from build123d import *

# Parameters (mm, degrees)
BOSS_EXTRUDE1_DEPTH = 59.69
SKETCH31_R          = 3.9878
CUT_EXTRUDE1_DEPTH  = 31.226


with BuildPart() as part:
    # Sketch30 → Boss-Extrude1 (new body)
    with BuildSketch(Plane(origin=(0, 0, -44.196), x_dir=(-1, 0, 0), z_dir=(0, 0, -1))):
        with BuildLine():
            Line((-21.122639806, -11.230837818), (-19.351377941, -18.999086285))
            Line((-19.351377941, -18.999086285), (-11.19917043, -18.999086285))
            Line((-11.19917043, -18.999086285), (-11.58017043, -47.00394942))
            Line((-11.58017043, -47.00394942), (-17.42217043, -47.00394942))
            Line((-17.42217043, -47.00394942), (-17.42217043, -26.68394942))
            Line((-17.42217043, -26.68394942), (-17.42217043, -25.349086285))
            ThreePointArc((-17.42217043, -25.349086285), (-25.786020569, -21.520936424), (-29.61417043, -13.157086285))
            Line((-29.61417043, -13.157086285), (-29.61417043, 6.33605058))
            ThreePointArc((-29.61417043, 6.33605058), (-25.894426551, 15.316306701), (-16.91417043, 19.03605058))
            Line((-16.91417043, 19.03605058), (0.10382957, 19.03605058))
            ThreePointArc((0.10382957, 19.03605058), (9.084085691, 15.316306701), (12.80382957, 6.33605058))
            Line((12.80382957, 6.33605058), (12.80382957, -13.157086285))
            ThreePointArc((12.80382957, -13.157086285), (8.975679709, -21.520936424), (0.61182957, -25.349086285))
            Line((0.61182957, -25.349086285), (0.61182957, -26.68394942))
            Line((0.61182957, -26.68394942), (0.61182957, -47.00394942))
            Line((0.61182957, -47.00394942), (-5.23017043, -47.00394942))
            Line((-5.23017043, -47.00394942), (-5.61117043, -18.999086285))
            Line((-5.61117043, -18.999086285), (2.54103708, -18.999086285))
            Line((2.54103708, -18.999086285), (4.312298946, -11.230837818))
            ThreePointArc((4.312298946, -11.230837818), (8.246380302, -8.403768679), (6.679296605, -3.81971319))
            ThreePointArc((6.679296605, -3.81971319), (7.525853874, 2.546365897), (5.417372104, 8.61249537))
            ThreePointArc((5.417372104, 8.61249537), (4.777900298, 13.775697179), (-0.415899, 14.079054992))
            ThreePointArc((-0.415899, 14.079054992), (-8.40517043, 15.22605058), (-16.394441861, 14.079054992))
            ThreePointArc((-16.394441861, 14.079054992), (-21.588241548, 13.775696815), (-22.227712388, 8.612494473))
            ThreePointArc((-22.227712388, 8.612494473), (-24.336184911, 2.546364848), (-23.489636452, -3.819712493))
            ThreePointArc((-23.489636452, -3.819712493), (-25.056721349, -8.403768093), (-21.122639806, -11.230837818))
        make_face()
    extrude(amount=BOSS_EXTRUDE1_DEPTH)

    # Sketch31 → Cut-Extrude1 (cut, through all)
    with BuildSketch(Plane(origin=(17.42217043, 0, 0), x_dir=(0, 0, -1), z_dir=(1, 0, 0))):
        with Locations(Location((95.9104, -36.00574942, 0), (0, 0, 90))):  # turned: the seam where the file's is
            Circle(SKETCH31_R)
        with Locations(Location((70.8914, -36.00574942, 0), (0, 0, 90))):  # turned: the seam where the file's is
            Circle(SKETCH31_R)
        with Locations(Location((54.1782, -38.11394942, 0), (0, 0, 90))):  # turned: the seam where the file's is
            Circle(SKETCH31_R)
    extrude(amount=-CUT_EXTRUDE1_DEPTH, mode=Mode.SUBTRACT)


solid = part.part
The model under review builds one solid part; all positions refer to its coordinate system, in mm. A direction names the side the tool comes from. Coordinates: 2 decimals unless noted, no trailing zeros. Loops run counter-clockwise (first coordinate to the right, second up) from the corner with the lowest first, then second, coordinate; pieces in that order, holes last. Notation, with made-up numbers: (-21.5, -0.5) -> (10.5, -0.5) arc R19 cw to (10.5, 15.5) -> close; hole circle Ø2 at (-19.75, -7.5). An arc over 180 degrees is marked (long way). Use a Markdown table: item, result. Add a question column.
1. To check wall thickness, follow line 1 (X direction, y = -35.5, z = -78.5); line 2 (Y direction, x = 12, z = -98); line 3 (Y direction, x = 22.5, z = -66). State the ranges of each line that lie inside material, in increasing order.
2. Draft analysis for pull direction Y (two halves, no side actions). For faces 1 (the face through (25.99, 15.22, -73.62)), 2 (the face through (-9.068, -21.427, -73.623)), 3 (the face through (2.439, -38.633, -50.224)), state which applies: pulls with the +Y half, pulls with the -Y half, needs draft (parallel to the pull), parting line crosses it, or undercut.
3. Add section D-D on x = 3. Write out the cut boundary in (y, z), plus the area to 3 significant figures.
4. Add section B-B on y = -9.5. Write out the cut boundary in (x, z), plus the area to 3 significant figures.
5. Add section C-C on z = -51. Give the number of separate pieces and of enclosed holes in the cut face, plus the area to 3 significant figures.
6. Machinability: for faces 4 (the face through (-8.224, -8.473, -73.623)), 5 (the face through (29.614, -4, -74)), 6 (the face through (-0.612, -31, -74)), which of the approach directions +Z, -Z, +X, -X, +Y, -Y give a long, thin tool a straight path to every point of the face, cutting with its end or side? Answer none if there is none.
7. Add section A-A on x = 12.5. Write out the cut boundary in (y, z), plus the area to 3 significant figures.
8. Clearance check with flat-ended pins moving along their axes: pin 1 Ø7 at (y, z) = (-38.11, -54.18) entering from -X; pin 2 Ø11 at (y, z) = (-40.5, -84.5) entering from +X; pin 3 Ø8 at (x, z) = (-5, -86.5) entering from -Y; pin 4 Ø5 at (y, z) = (-38.5, -58) entering from -X. State where each tip first meets the part, or that it passes through.
Returned:
| question | item | result |
|---|---|---|
| 1 | line 1 | x = -0.61 to 5.39, 11.42 to 17.42 |
| 1 | line 2 | y = -47 to -39.4, -32.61 to -19, 15 to 19.04 |
| 1 | line 3 | y = -23.92 to -11.01, 8.17 to 9.11, 12.51 to 17.74 |
| 2 | face 1 | pulls with the +Y half |
| 2 | face 2 | pulls with the -Y half |
| 2 | face 3 | undercut |
| 3 | outline | (-47, -103.89) -> (-19, -103.89) -> (-19, -44.2) -> (-47, -44.2) -> close; (14.71, -103.89) -> (19.04, -103.89) -> (19.04, -44.2) -> (14.71, -44.2) -> close; hole circle Ø7.98 at (-38.11, -54.18); hole circle Ø7.98 at (-36.01, -95.91); hole circle Ø7.98 at (-36.01, -70.89) |
| 3 | area | 1,780 mm² |
| 4 | outline | (-12.8, -103.89) -> (-7.7, -103.89) -> (-7.7, -44.2) -> (-12.8, -44.2) -> close; (24.51, -103.89) -> (29.61, -103.89) -> (29.61, -44.2) -> (24.51, -44.2) -> close |
| 4 | area | 609 mm² |
| 5 | separate pieces | 3 |
| 5 | enclosed holes | 0 |
| 5 | area | 928 mm² |
| 6 | face 4 | +Z, -Z |
| 6 | face 5 | +Z, -Z, +X, +Y, -Y |
| 6 | face 6 | +Z, -Z, -X, -Y |
| 7 | outline | (-47, -103.89) -> (-19, -103.89) -> (-19, -44.2) -> (-47, -44.2) -> close; (14.93, -103.89) -> (19.04, -103.89) -> (19.04, -44.2) -> (14.93, -44.2) -> close; hole circle Ø7.98 at (-38.11, -54.18); hole circle Ø7.98 at (-36.01, -95.91); hole circle Ø7.98 at (-36.01, -70.89) |
| 7 | area | 1,770 mm² |
| 8 | pin 1 | passes through |
| 8 | pin 2 | stops at x = 17.42 |
| 8 | pin 3 | stops at y = -25.31 |
| 8 | pin 4 | stops at x = -0.61 |
